Can you work these out from the model? Positions are in its coordinate system, mm. Face numbers are marked on the shaded views. A direction names the side the tool comes from. Give positions to 0.01 mm unless a question says otherwise; leave off trailing zeros. Loops run counter-clockwise (first coordinate to the right, second up) from the corner with the lowest first, then second, coordinate; pieces in that order, holes last. Notation, with made-up numbers: M 85.25,8 L 125.25,8 A15 ccw 125.25,16 Z; hole C 17,-40 d10. An arc over 180 degrees is marked long. Use CSV: the item, a comma, the result in double quotes.
from build123d import *

# Parameters (mm, degrees)
BOSS_EXTRUDE1_DEPTH = 60
SKETCH3_W           = 50
SKETCH3_H           = 57.5
CUT_EXTRUDE6_DEPTH  = 80
SKETCH9_R           = 5
CUT_EXTRUDE7_DEPTH  = 80
SKETCH10_W          = 61.517068372
SKETCH10_H          = 50
CUT_EXTRUDE8_DEPTH  = 62.5
SKETCH13_R          = 1.5
CUT_EXTRUDE9_DEPTH  = 131.227197428


with BuildPart() as part:
    # Sketch1 → Boss-Extrude1 (new body)
    with BuildSketch(Plane.XY):
        Polygon((97.225886213, 0), (47.225886213, 0), (0, -29.989383259), (0, -80), (97.225886213, -80), align=None)
    extrude(amount=BOSS_EXTRUDE1_DEPTH)

    # Sketch3 → Cut-Extrude6 (cut)
    with BuildSketch(Plane.ZY):
        with Locations((30, -33.75)):
            Rectangle(SKETCH3_W, SKETCH3_H)
    extrude(amount=-CUT_EXTRUDE6_DEPTH, mode=Mode.SUBTRACT)

    # Sketch9 → Cut-Extrude7 (cut)
    with BuildSketch(Plane.ZY.offset(-80)):
        with Locations(Location((30, -41.5, 0), (0, 0, 270))):
            Circle(SKETCH9_R)
    extrude(amount=-CUT_EXTRUDE7_DEPTH, mode=Mode.SUBTRACT)

    # Sketch10 → Cut-Extrude8 (cut)
    with BuildSketch(Plane(origin=(0, 0, 0), x_dir=(1, 0, 0), z_dir=(0, 1, 0))):
        with Locations((61.467352027, -30)):
            Rectangle(SKETCH10_W, SKETCH10_H)
    extrude(amount=-CUT_EXTRUDE8_DEPTH, mode=Mode.SUBTRACT)

    # Sketch13 → Cut-Extrude9 (cut, through all)
    with BuildSketch(Plane(origin=(0, -62.5, 0), x_dir=(1, 0, 0), z_dir=(0, 1, 0))):
        with Locations(Location((10, -15, 0), (0, 0, 180))):
            Circle(SKETCH13_R)
        with Locations(Location((82.225886213, -15, 0), (0, 0, 180))):
            Circle(SKETCH13_R)
        with Locations(Location((10, -45, 0), (0, 0, 180))):
            Circle(SKETCH13_R)
        with Locations(Location((82.225886213, -45, 0), (0, 0, 180))):
            Circle(SKETCH13_R)
    extrude(amount=-CUT_EXTRUDE9_DEPTH, mode=Mode.SUBTRACT)


solid = part.part
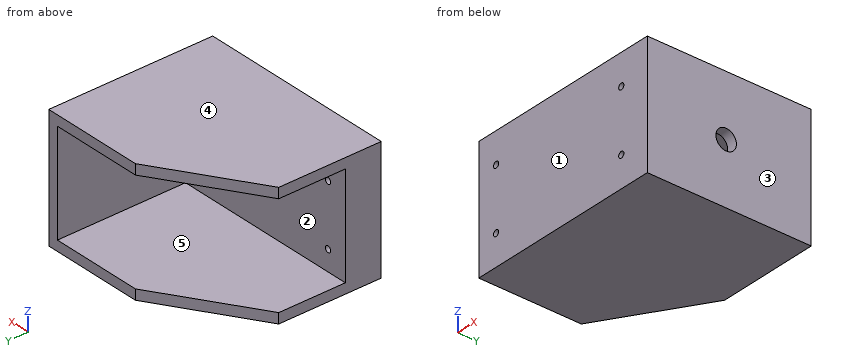
Q1. I'm going to push flat-ended pins straight in: P1, Ø2.5, axis at x = 10, z = 15, coming from the +Y side; P2, Ø4, axis at x = 60, z = 46.5, coming from the +Y side; P3, Ø25, axis at y = -31, z = 19, coming from the -X side. Where does each tip first touch, or does it pass through?
Model answer:
P1,"through"
P2,"y = -62.5"
P3,"x = 92.23"
Q2. Please list where these lines run through material, in increasing order: L1, parallel to Z at x = 10, y = -75.5; L2, parallel to Z at x = 38, y = -21; L3, parallel to Z at x = 96.25, y = -41.5. Write a range as from..to.
Model answer:
L1,"0..13.5, 16.5..43.5, 46.5..60"
L2,"0..5, 55..60"
L3,"0..25, 35..60"
Q3. I want a section at D-D, the plane y = -60. Please give me the cut outline in (x, z), then the cut area to 3 significant figures.
Model answer:
outline,"M 0,0 L 97.23,0 L 97.23,60 L 0,60 L 0,55 L 92.23,55 L 92.23,5 L 0,5 Z"
area,"1,220 mm2"
Q4. I want a section at C-C, the plane z = 30. Please give me the cut outline in (x, y).
Model answer:
outline,"M 0,-80 L 97.23,-80 L 97.23,-46.5 L 92.23,-46.5 L 92.23,-62.5 L 0,-62.5 Z; M 92.23,-36.5 L 97.23,-36.5 L 97.23,0 L 92.23,0 Z"
Q5. If we mould it in two halves opening along Z, with no side actions, what happens to the marked faces 3, 4 and 5? For each: released by +Z, released by -Z, zero draft, split by the parting line, or undercut.
Model answer:
face 3,"zero draft"
face 4,"released by +Z"
face 5,"undercut"
Q6. For the marked faces 1 and 2, which set-ups out of +Z, -Z, +X, -X, +Y, -Y let a thin tool reach every point of the face, with its end or its side?
Model answer:
face 1,"+Z, -Z, +X, -X, -Y"
face 2,"-X, +Y"
Q7. I want a section at B-B, the plane y = -41.5. Please give me the cut outline in (x, z).
Model answer:
outline,"M 0,0 L 97.23,0 L 97.23,25 L 92.23,25 L 92.23,5 L 0,5 Z; M 0,55 L 92.23,55 L 92.23,35 L 97.23,35 L 97.23,60 L 0,60 Z"
Q8. I want a section at A-A, the plane z = 15. Please give me the cut outline in (x, y).
Model answer:
outline,"M 0,-80 L 8.5,-80 L 8.5,-62.5 L 0,-62.5 Z; M 11.5,-80 L 80.73,-80 L 80.73,-62.5 L 11.5,-62.5 Z; M 83.73,-80 L 97.23,-80 L 97.23,0 L 92.23,0 L 92.23,-62.5 L 83.73,-62.5 Z"
